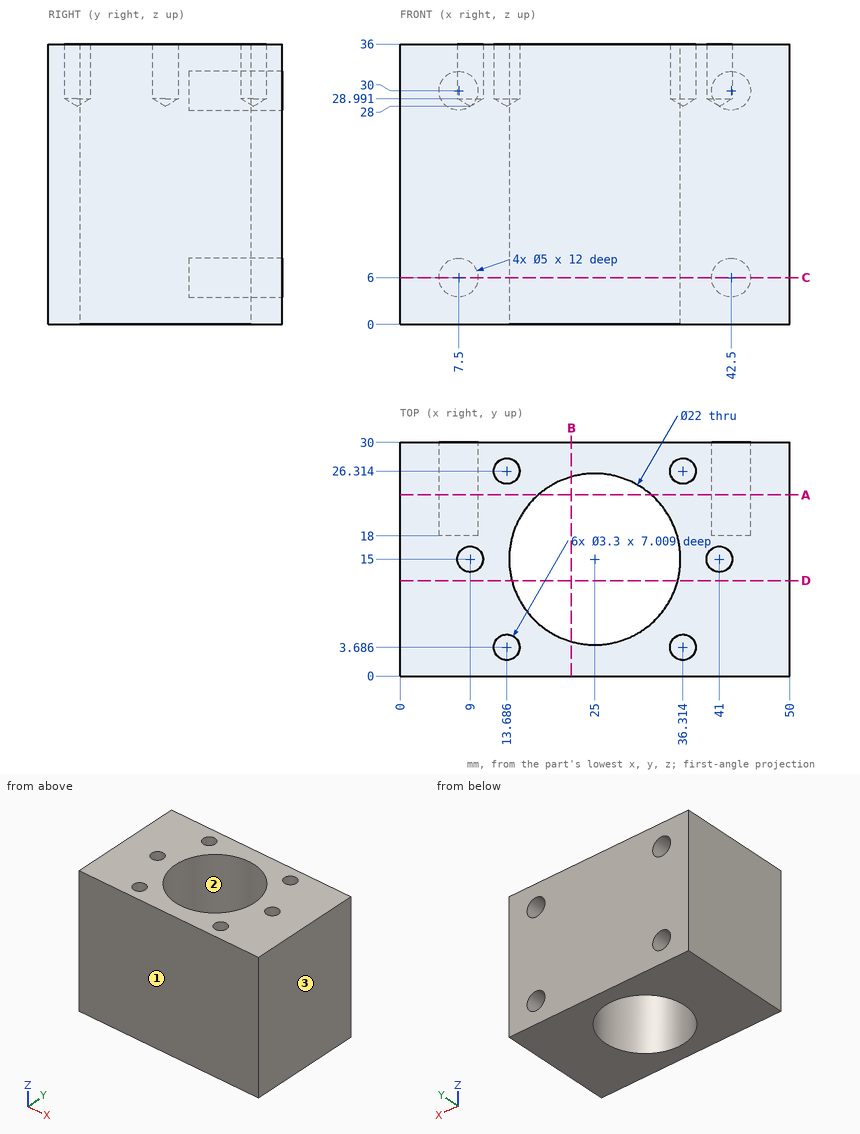
Job drawing, mm, ordinate dimensions from the low corner. One solid piece. Round coordinates to 2 decimals unless told otherwise and drop trailing zeros. Loops run counter-clockwise (first coordinate to the right, second up) from the corner with the lowest first, then second, coordinate; pieces in that order, holes last. Notation, with made-up numbers: (25.25, 2.25) -> (50.25, 2.25) arc R34 ccw to (50.25, 39.25) -> close; hole circle Ø2 at (84, 85.25). An arc over 180 degrees is marked (long way). One line per item, written item: value. Start each with the question number.
Q1. Cut at B-B on x = 22. List the corners of the cut face in (y, z).
Q2. Cut at D-D on y = 12.25. List the corners of the cut face in (x, z).
Q3. Cut at A-A on y = 23.25. List the corners of the cut face in (x, z) (1 decimal), plus the area to 3 significant figures.
Q4. Two-plate mould, pull along X, no slides. Class the marked faces 1, 2 and 3: released by +X, released by -X, zero draft, split by the parting line, or undercut.
Q5. Cut at C-C on z = 6. List the corners of the cut face in (x, y).
Q6. Drop flat-ended pins along their axis: pin 1 Ø4.5 at (x, z) = (7.5, 6) entering from +Y; pin 2 Ø2 at (x, y) = (13.69, 3.69) entering from +Z (1 decimal). Give the stop position or say it passes through.
Q7. Probe line 1 along Y through (x, z) = (13.5, 34) (1 decimal); line 2 along Y through (x, z) = (24.5, 6.5); line 3 along X through (y, z) = (9, 11). List the from-to ranges inside material, lowest first.
Computed:
1. outline: (0, 0) -> (4.42, 0) -> (4.42, 36) -> (0, 36) -> close; (25.58, 0) -> (30, 0) -> (30, 36) -> (25.58, 36) -> close
2. outline: (0, 0) -> (14.35, 0) -> (14.35, 36) -> (0, 36) -> close; (35.65, 0) -> (50, 0) -> (50, 36) -> (35.65, 36) -> close
3. outline: (0, 0) -> (17.7, 0) -> (17.7, 36) -> (0, 36) -> close; (32.3, 0) -> (50, 0) -> (50, 36) -> (32.3, 36) -> close; hole circle Ø5 at (7.5, 6); hole circle Ø5 at (7.5, 30); hole circle Ø5 at (42.5, 6); hole circle Ø5 at (42.5, 30)
3. area: 1,200 mm²
4. face 1: zero draft
4. face 2: undercut
4. face 3: released by +X
5. outline: (0, 0) -> (50, 0) -> (50, 30) -> (45, 30) -> (45, 18) -> (40, 18) -> (40, 30) -> (10, 30) -> (10, 18) -> (5, 18) -> (5, 30) -> (0, 30) -> close; hole circle Ø22 at (25, 15)
6. pin 1: y = 18
6. pin 2: z = 28.6
7. line 1: 0 to 2, 5.3 to 24.7, 28 to 30
7. line 2: 0 to 4.01, 25.99 to 30
7. line 3: 0 to 15.78, 34.22 to 50
